Part print with two shaded views. Sizes in mm from the minimum x, y, z corner. Coordinates: 2 decimals unless noted, no trailing zeros. Order: outer loops, then holes, each group sorted by start corner. A loop starts at its lowest first (then second) coordinate and runs counter-clockwise, first axis right, second up. Notation, with made-up numbers: (39.5, 11.5) - (69.5, 11.5) arc R17 ccw to (69.5, 23.5) - close; hole circle Ø3 at (54.5, 54). An arc over 180 degrees is marked (long way). One line per item, written item: value.
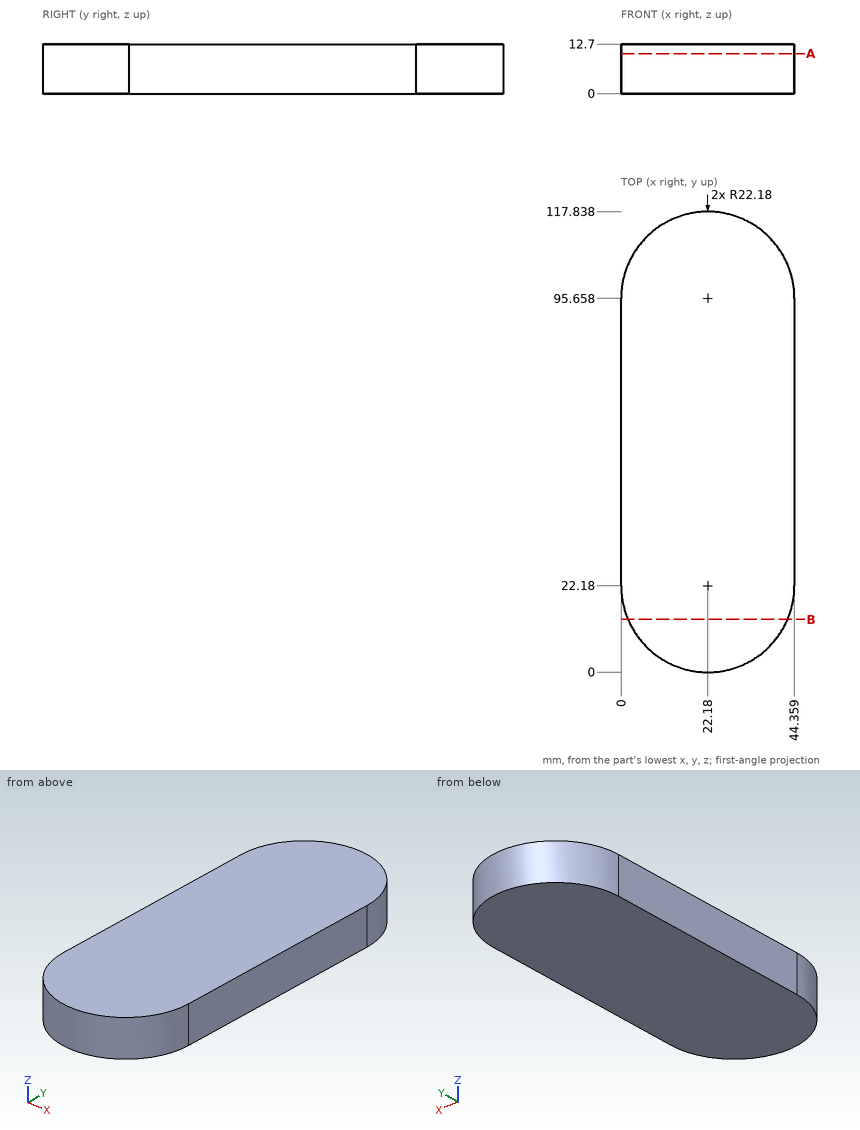
1. Band-saw the part on B-B, the plane y = 13.5. Give the cut face in (x, z).
Values found:
outline: (1.77, 0) - (42.59, 0) - (42.59, 12.7) - (1.77, 12.7) - close
2. Flat gauge pins, fed straight in: P1, Ø6, axis at x = 19.5, z = 5, coming from the +Y side; P2, Ø3, axis at x = 16, z = 10.5, coming from the +Y side; P3, Ø1, axis at x = 17.5, z = 1.5, coming from the +Y side. Where does each tip first touch, or does it go through?
Values found:
P1: stops at y = 117.84
P2: stops at y = 117.34
P3: stops at y = 117.44
3. Band-saw the part on A-A, the plane z = 10.25. Give the cut face in (x, y), and give its area (4 significant figures).
Values found:
outline: (0, 22.18) arc R22.18 ccw to (44.36, 22.18) - (44.36, 95.66) arc R22.18 ccw to (0, 95.66) - close
area: 4,805 mm2
4. Probe line 1 along Y through (x, z) = (23, 8) (1 decimal); line 2 along Y through (x, z) = (8, 8.75) (1 decimal); line 3 along X through (y, z) = (9.5, 3.25). List the from-to ranges inside material, lowest first.
Values found:
line 1: y = 0 to 117.8
line 2: y = 5.1 to 112.7
line 3: x = 3.98 to 40.38
